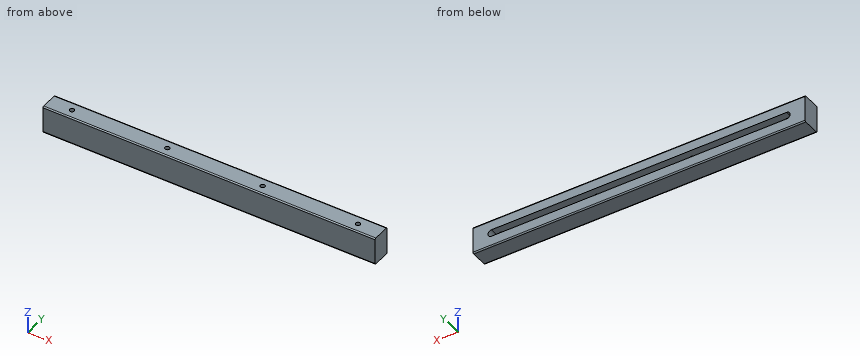
```python
from build123d import *

# Parameters (mm, degrees)
F0_W     = 914.4
F0_H     = 76.2
F1_DEPTH = 50.8
F2_R     = 6.35
F3_DEPTH = 47.625
F5_DEPTH = 25.4
F7_DEPTH = 914.401


with BuildPart() as f1:
    # F0 (on Front) → F1 (new body)
    with BuildSketch(Plane.XZ):
        Rectangle(F0_W, F0_H)
    extrude(amount=F1_DEPTH)

    # F2 (on face) → F3 (cut)
    with BuildSketch(Plane.XY.offset(38.1)):
        with Locations((-393.7, -25.4)):
            Circle(F2_R)
        with Locations((393.7, -25.4)):
            Circle(F2_R)
        with Locations((-131.318, -25.4)):
            Circle(F2_R)
        with Locations((131.318, -25.4)):
            Circle(F2_R)
    extrude(amount=-F3_DEPTH, mode=Mode.SUBTRACT)

    # F4 (on face) → F5 (cut)
    with BuildSketch(Plane(origin=(0, 0, 0), x_dir=(-1, 0, 0), z_dir=(0, 1, 0))):
        with BuildLine():
            Line((405.930353, 9.525), (-406.4, 9.525))
            ThreePointArc((-406.4, 9.525), (-415.922103, -0.234895), (-405.930353, -9.513415))
            Line((-405.930353, -9.513415), (406.4, -9.513415))
            ThreePointArc((406.4, -9.513415), (415.922103, 0.24648), (405.930353, 9.525))
        make_face()
    extrude(amount=-F5_DEPTH, mode=Mode.SUBTRACT)

    # F6 (on face) → F7 (cut, through all)
    with BuildSketch(Plane(origin=(-457.2, 0, 0), x_dir=(0, -1, 0), z_dir=(-1, 0, 0))):
        with BuildLine():
            ThreePointArc((0, 34.925), (0.929936, 37.170064), (3.175, 38.1))
            Line((3.175, 38.1), (0, 38.1))
            Line((0, 38.1), (0, 34.925))
        make_face()
        with BuildLine():
            ThreePointArc((47.625, 38.1), (49.870064, 37.170064), (50.8, 34.925))
            Line((50.8, 34.925), (50.8, 38.1))
            Line((50.8, 38.1), (47.625, 38.1))
        make_face()
        with BuildLine():
            ThreePointArc((3.175, -38.1), (0.929936, -37.170064), (0, -34.925))
            Line((0, -34.925), (0, -38.1))
            Line((0, -38.1), (3.175, -38.1))
        make_face()
        with BuildLine():
            ThreePointArc((50.8, -34.925), (49.870064, -37.170064), (47.625, -38.1))
            Line((47.625, -38.1), (50.8, -38.1))
            Line((50.8, -38.1), (50.8, -34.925))
        make_face()
    extrude(amount=-F7_DEPTH, mode=Mode.SUBTRACT)


solid = f1.part
```
Work out the finished part from the listing and answer in its coordinate system (mm). Coordinates: 2 decimals unless noted, no trailing zeros. Loops run counter-clockwise (first coordinate to the right, second up) from the corner with the lowest first, then second, coordinate; pieces in that order, holes last. Notation, with made-up numbers: M 54.25,27 L 64.25,27 A29 cw 64.25,53 Z; hole C 28,17 d4. An arc over 180 degrees is marked long. Use CSV: the item, a comma, the result in double quotes. Start each with the question number.
(1) Find section A-A, the plane x = -215. Give the vertices of the cut face in (y, z) (3 decimals).
(2) Find section B-B, the plane z = 0. Give the vertices of the cut face in (x, y) (3 decimals), then the cut area to 3 significant figures.
(3) Given pin 1 Ø7.5 at (x, y) = (-131.318, -25.4) entering from +Z (3 decimals); pin 2 Ø14 at (x, y) = (134.5, -26) entering from +Z; pin 3 Ø15 at (x, z) = (30.5, -1) entering from +Y, each flat-ended and moving along its own axis, determine where each tip first touches the part or whether it passes through.
(4) Consider line 1 (X direction, y = -25.4, z = 24); line 2 (Y direction, x = -393, z = 28); line 3 (Z direction, x = 42.5, y = -7.5) (3 decimals). Determine where each line is inside the solid, lowest interval first.
Recorded:
1,outline,"M -50.8,-34.925 A3.175 ccw -47.625,-38.1 L -3.175,-38.1 A3.175 ccw 0,-34.925 L 0,-9.513 L -25.4,-9.513 L -25.4,9.525 L 0,9.525 L 0,34.925 A3.175 ccw -3.175,38.1 L -47.625,38.1 A3.175 ccw -50.8,34.925 Z"
2,outline,"M -457.2,-50.8 L 457.2,-50.8 L 457.2,0 L 415.925,0 L 415.925,-25.4 L 400.05,-25.4 A6.35 cw 387.35,-25.4 L 137.668,-25.4 A6.35 cw 124.968,-25.4 L -124.968,-25.4 A6.35 cw -137.668,-25.4 L -387.35,-25.4 A6.35 cw -400.05,-25.4 L -415.925,-25.4 L -415.925,0 L -457.2,0 Z"
2,area,"25,100 mm^2"
3,pin 1,"stops at z = -9.525"
3,pin 2,"stops at z = 38.1"
3,pin 3,"stops at y = -25.4"
4,line 1,"x = -457.2 to -400.05, -387.35 to -137.67, -124.97 to 124.97, 137.67 to 387.35, 400.05 to 457.2"
4,line 2,"y = -50.8 to -31.71, -19.09 to 0"
4,line 3,"z = -38.1 to -9.513, 9.525 to 38.1"
